from build123d import *

# Parameters (mm, degrees)
F1_DEPTH = 12
F2_W     = 13
F2_H     = 4
F3_DEPTH = 8
F4_DEPTH = 25
F6_DEPTH = 5


with BuildPart() as f1:
    # F0 (on Top) → F1 (new body)
    with BuildSketch(Plane.XY):
        with BuildLine():
            Line((64, 72.6), (-61, 72.6))
            ThreePointArc((-61, 72.6), (-66.656854, 70.256854), (-69, 64.6))
            Line((-69, 64.6), (-69, -60.4))
            ThreePointArc((-69, -60.4), (-66.656854, -66.056855), (-61, -68.4))
            Line((-61, -68.4), (64, -68.4))
            ThreePointArc((64, -68.4), (69.656854, -66.056855), (72, -60.4))
            Line((72, -60.4), (72, 64.6))
            ThreePointArc((72, 64.6), (69.656854, 70.256854), (64, 72.6))
        make_face()
        with BuildLine():
            Line((64, -64.4), (-61, -64.4))
            ThreePointArc((-61, -64.4), (-63.828427, -63.228428), (-65, -60.4))
            Line((-65, -60.4), (-65, 64.6))
            ThreePointArc((-65, 64.6), (-63.828427, 67.428427), (-61, 68.6))
            Line((-61, 68.6), (64, 68.6))
            ThreePointArc((64, 68.6), (66.828427, 67.428427), (68, 64.6))
            Line((68, 64.6), (68, -60.4))
            ThreePointArc((68, -60.4), (66.828427, -63.228428), (64, -64.4))
        make_face(mode=Mode.SUBTRACT)
    extrude(amount=F1_DEPTH)

    # F2 (on face) → F3 (join)
    with BuildSketch(Plane.XZ.offset(-68.6)):
        Polygon((-48, 12), (-48, 6), (-48, 0), (-47.4, 0), (-47.4, 5), (-41.2, 5), (-41.2, 0), (-40.6, 0), (-40.6, 5), (-33.6, 5), (-33.6, 0), (-33, 0), (-33, 12), align=None)
        with Locations((-40.5, 8)):
            Rectangle(F2_W, F2_H, mode=Mode.SUBTRACT)
        Polygon((9, 12), (-6, 12), (-6, 6), (-6, 0), (-5.4, 0), (-5.4, 5), (0.9, 5), (0.9, 0), (1.5, 0), (1.5, 5), (8.4, 5), (8.4, 0), (9, 0), align=None)
        with Locations((1.5, 8)):
            Rectangle(F2_W, F2_H, mode=Mode.SUBTRACT)
        Polygon((51, 12), (36, 12), (36, 0), (36.6, 0), (36.6, 5), (42.9, 5), (42.9, 0), (43.5, 0), (43.5, 5), (50.4, 5), (50.4, 0), (51, 0), (51, 6), align=None)
        with Locations((43.5, 8)):
            Rectangle(F2_W, F2_H, mode=Mode.SUBTRACT)
    extrude(amount=-F3_DEPTH)

    # F2 (on face) → F4 (cut)
    with BuildSketch(Plane.XZ.offset(-68.6)):
        with Locations((43.5, 8)):
            Rectangle(F2_W, F2_H)
        with Locations((1.5, 8)):
            Rectangle(F2_W, F2_H)
        with Locations((-40.5, 8)):
            Rectangle(F2_W, F2_H)
    extrude(amount=-F4_DEPTH, mode=Mode.SUBTRACT)

    # F5 (on face) → F6 (join)
    with BuildSketch(Plane(origin=(0, -64.4, 0), x_dir=(-1, 0, 0), z_dir=(0, 1, 0))):
        Polygon((-18.5, 4), (-18.5, 12), (-21, 12), (-21, 6.5), (-37, 6.5), (-37, 12), (-39.5, 12), (-39.5, 4), (-39.5, 0), (-38.9, 0), (-38.9, 4), (-29.7, 4), (-29.7, 0), (-29.1, 0), (-29.1, 4), (-19.1, 4), (-19.1, 0), (-18.5, 0), align=None)
        Polygon((18, 12), (15.5, 12), (15.5, 4), (15.5, 0), (16.1, 0), (16.1, 4), (24.702823, 4), (24.702823, 0), (25.302823, 0), (25.302823, 4), (35.9, 4), (35.9, 0), (36.5, 0), (36.5, 4), (36.5, 12), (34, 12), (34, 6.5), (18, 6.5), align=None)
    extrude(amount=F6_DEPTH)


solid = f1.part
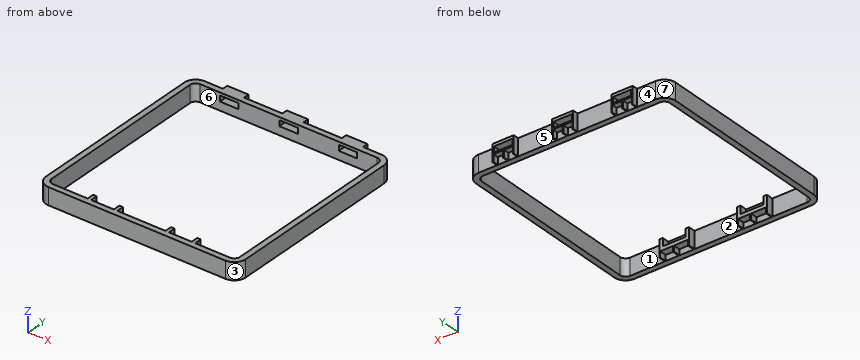
Design review of the part built by this model. Coordinates are the model's own, in mm. Face numbers are marked on the shaded views. A direction names the side the tool comes from. Coordinates: 2 decimals unless noted, no trailing zeros. Loops run counter-clockwise (first coordinate to the right, second up) from the corner with the lowest first, then second, coordinate; pieces in that order, holes last. Notation, with made-up numbers: (-17.5, 44) - (23.5, 44) arc R11 ccw to (23.5, 50) - close; hole circle Ø11 at (88, 59.5). An arc over 180 degrees is marked (long way). Use CSV: the item, a comma, the result in double quotes. Start each with the question number.
1. Clearance check with flat-ended pins moving along their axes: pin 1 (2 mm diameter, centred on y = 75.5, z = 1.5, fed in from +X); pin 2 (3.5 mm diameter, centred on x = 58.5, z = 4.5, fed in from +Y); pin 3 (2.5 mm diameter, centred on y = -62.5, z = 9.5, fed in from +X). State where each tip first meets the part, or that it passes through.
2. Mouldability with a two-part tool opening along Y and no side actions: class the marked faces 1, 2, 3 and 4 as released by +Y, released by -Y, zero draft, split by the parting line, or undercut.
3. Add section A-A on x = 15.5. Give the boundary of the cut face in (y, z).
4. Add section B-B on y = 14. Give the boundary of the cut face in (x, z), plus the area to 3 significant figures.
5. Add section D-D on z = 8.25. Count the separate pieces of the cut face and the enclosed holes in it, plus the area to 3 significant figures.
6. Add section C-C on x = -44. Give the boundary of the cut face in (y, z), plus the area to 3 significant figures.
7. For the marked faces 5, 6 and 7, list the 3-axis set-ups (+Z, -Z, +X, -X, +Y, -Y) from which the entire face can be reached by the end or side of a thin tool; tool diameter is ignored.
8. To check wall thickness, follow probe 1 along Y at (x, z) = (61, 10.5); probe 2 along X at (y, z) = (-21, 8.75); probe 3 along Y at (x, z) = (50.5, 4). State the ranges of each line that lie inside material, in increasing order.
Resolved:
1,pin 1,"x = 51"
1,pin 2,"y = 72.6"
1,pin 3,"x = 71.95"
2,face 1,"undercut"
2,face 2,"undercut"
2,face 3,"released by -Y"
2,face 4,"released by +Y"
3,outline,"(-68.4, 0) - (-64.4, 0) - (-64.4, 12) - (-68.4, 12) - close; (68.6, 0) - (72.6, 0) - (72.6, 12) - (68.6, 12) - close"
4,outline,"(-69, 0) - (-65, 0) - (-65, 12) - (-69, 12) - close; (68, 0) - (72, 0) - (72, 12) - (68, 12) - close"
4,area,"96.0 mm2"
5,separate pieces,"3"
5,enclosed holes,"0"
5,area,"2,070 mm2"
6,outline,"(-68.4, 0) - (-64.4, 0) - (-64.4, 12) - (-68.4, 12) - close; (68.6, 0) - (72.6, 0) - (72.6, 5) - (76.6, 5) - (76.6, 6) - (68.6, 6) - close; (68.6, 10) - (76.6, 10) - (76.6, 12) - (68.6, 12) - close"
6,area,"92.0 mm2"
7,face 5,"+Z, -Z, +Y"
7,face 6,"+Z, -Z"
7,face 7,"+Z, -Z, -X, +Y"
8,probe 1,"-68.4 to -64.4, 68.6 to 72.6"
8,probe 2,"-69 to -65, 68 to 72"
8,probe 3,"-68.4 to -64.4, 68.6 to 76.6"
